For this review, take the finished solid that the model builds, in its own axes (mm). Coordinates: 2 decimals unless noted, no trailing zeros. Write each loop counter-clockwise with the first axis right and the second up, starting at its lowest first coordinate (ties: lowest second). Pieces come first, ordered by that corner, then holes.
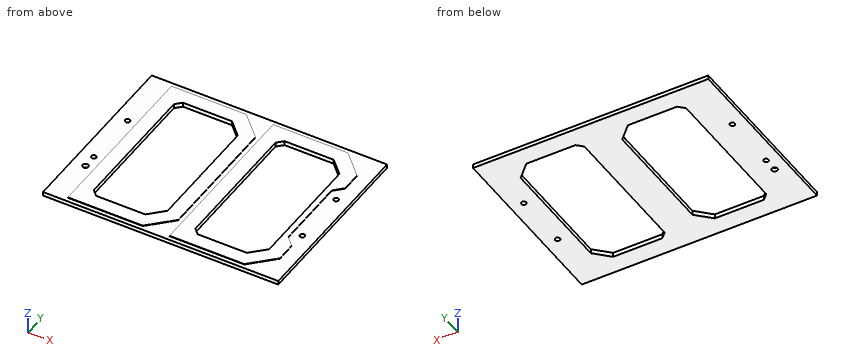
```python
from build123d import *

# Parameters (mm, degrees)
SKETCH1_W           = 105.41
SKETCH1_H           = 82
SKETCH1_R           = 1.0795
SKETCH1_R_2         = 1.27
BOSS_EXTRUDE1_DEPTH = 1.778
BOSS_EXTRUDE2_DEPTH = 0.2
CUT_EXTRUDE1_DEPTH  = 2.978
CHAMFER1_SIZE       = 2.54


with BuildPart() as part:
    # Sketch1 → Boss-Extrude1 (new body)
    with BuildSketch(Plane.XY):
        Rectangle(SKETCH1_W, SKETCH1_H)
        with Locations((46.7106, 12.7)):
            Circle(SKETCH1_R, mode=Mode.SUBTRACT)
        with Locations((46.7106, -12.7)):
            Circle(SKETCH1_R, mode=Mode.SUBTRACT)
        with Locations((-46.7106, 12.7)):
            Circle(SKETCH1_R, mode=Mode.SUBTRACT)
        with Locations((-46.7106, -12.7)):
            Circle(SKETCH1_R, mode=Mode.SUBTRACT)
        with Locations((-46.7106, -19.05)):
            Circle(SKETCH1_R_2, mode=Mode.SUBTRACT)
    extrude(amount=BOSS_EXTRUDE1_DEPTH)

    # Sketch2 → Boss-Extrude2 (add)
    with BuildSketch(Plane.XY.offset(1.778)):
        Polygon((-9.175, 39.095), (0.825, 29.095), (0.825, -29.095), (-9.175, -39.095), (-42.705, -39.095), (-42.705, 39.095), align=None)
        Polygon((46.355, 20.205), (42.545, 16.395), (42.545, -16.395), (46.355, -20.205), (46.355, -29.095), (36.355, -39.095), (2.825, -39.095), (2.825, 39.095), (36.355, 39.095), (46.355, 29.095), align=None)
    extrude(amount=BOSS_EXTRUDE2_DEPTH)

    # Sketch3 → Cut-Extrude1 (cut, through all)
    with BuildSketch(Plane.XY.offset(1.978)):
        Polygon((-36.355, -32.745), (-36.355, 32.745), (-11.805256121, 32.745), (-5.525, 26.464743879), (-5.525, -26.464743879), (-11.805256121, -32.745), align=None)
        Polygon((9.175, -32.745), (9.175, 32.745), (33.724743879, 32.745), (40.005, 26.464743879), (40.005, -26.464743879), (33.724743879, -32.745), align=None)
    extrude(amount=-CUT_EXTRUDE1_DEPTH, mode=Mode.SUBTRACT)

    # Chamfer1
    chamfer1_edges = [part.edges().sort_by_distance(p)[0] for p in [
        (-36.355, -32.745, 0.989),
        (-36.355, 32.745, 0.989),
        (9.175, -32.745, 0.989),
        (9.175, 32.745, 0.989),
    ]]
    chamfer(chamfer1_edges, length=CHAMFER1_SIZE)


solid = part.part
```
Q1. For probe 1 along X at (y, z) = (-8, 1.4) (3 decimals); probe 2 along X at (y, z) = (-23.5, 1.85) (3 decimals); probe 3 along Y at (x, z) = (-21.5, 0.6) (3 decimals), list the stretches that pass through material, from the lowest coordinate up.
Ans:
probe 1: x = -52.705 to -36.355, -5.525 to 9.175, 40.005 to 52.705
probe 2: x = -42.705 to -36.355, -5.525 to 0.825, 2.825 to 9.175, 40.005 to 46.355
probe 3: y = -41 to -32.745, 32.745 to 41
Q2. Add section C-C (z = 1.3). Give the number of separate pieces and of enclosed holes in the cut face, then the cut area to 3 significant figures.
Ans:
separate pieces: 1
enclosed holes: 7
area: 4,680 mm2
Q3. Add section A-A (y = -12.7). State the section outline as (x, z) points (3 decimals), then the cut area to 3 significant figures.
Ans:
outline: (-52.705, 0) - (-47.79, 0) - (-47.79, 1.778) - (-52.705, 1.778) - close; (-45.631, 0) - (-36.355, 0) - (-36.355, 1.978) - (-42.705, 1.978) - (-42.705, 1.778) - (-45.631, 1.778) - close; (-5.525, 0) - (9.175, 0) - (9.175, 1.978) - (2.825, 1.978) - (2.825, 1.778) - (0.825, 1.778) - (0.825, 1.978) - (-5.525, 1.978) - close; (40.005, 0) - (45.631, 0) - (45.631, 1.778) - (42.545, 1.778) - (42.545, 1.978) - (40.005, 1.978) - close; (47.79, 0) - (52.705, 0) - (52.705, 1.778) - (47.79, 1.778) - close
area: 74.4 mm2
Q4. Add section D-D (x = -27). State the section outline as (y, z) points (3 decimals).
Ans:
outline: (-41, 0) - (-32.745, 0) - (-32.745, 1.978) - (-39.095, 1.978) - (-39.095, 1.778) - (-41, 1.778) - close; (32.745, 0) - (41, 0) - (41, 1.778) - (39.095, 1.778) - (39.095, 1.978) - (32.745, 1.978) - close
Q5. Add section B-B (y = 18.5). State the section outline as (x, z) points (3 decimals).
Ans:
outline: (-52.705, 0) - (-36.355, 0) - (-36.355, 1.978) - (-42.705, 1.978) - (-42.705, 1.778) - (-52.705, 1.778) - close; (-5.525, 0) - (9.175, 0) - (9.175, 1.978) - (2.825, 1.978) - (2.825, 1.778) - (0.825, 1.778) - (0.825, 1.978) - (-5.525, 1.978) - close; (40.005, 0) - (52.705, 0) - (52.705, 1.778) - (44.65, 1.778) - (44.65, 1.978) - (40.005, 1.978) - close
Q6. Clearance check with flat-ended pins moving along their axes: pin 1 Ø3.5 at (x, y) = (-46.71, -19.05) entering from +Z; pin 2 Ø1.3 at (x, y) = (-46.71, -12.7) entering from +Z. State where each tip first meets the part, or that it passes through.
Ans:
pin 1: stops at z = 1.78
pin 2: passes through
